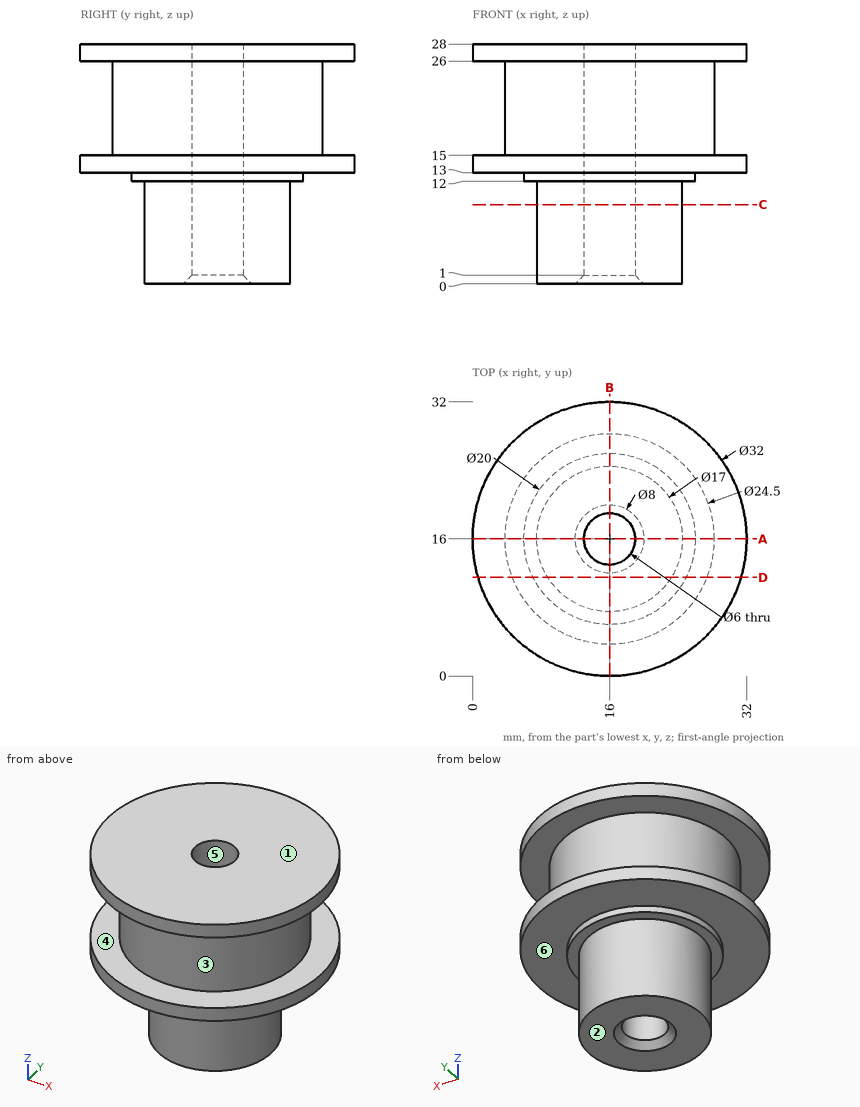
Part print with two shaded views. Sizes in mm from the minimum x, y, z corner. A direction names the side the tool comes from. Give positions to 0.01 mm unless a question says otherwise; leave off trailing zeros. Loops run counter-clockwise (first coordinate to the right, second up) from the corner with the lowest first, then second, coordinate; pieces in that order, holes last. Notation, with made-up numbers: (70, 19) - (78, 19) arc R25 cw to (78, 42) - close; hole circle Ø5 at (52, 23). An arc over 180 degrees is marked (long way). Put each result on its own line as item: value.
Q1. Mould opens along Z. For the marked faces 1, 2 and 3 say: pulls with the +Z half, pulls with the -Z half, needs draft (parallel to the pull), parting line crosses it, or undercut.
Filled in:
face 1: pulls with the +Z half
face 2: pulls with the -Z half
face 3: undercut
Q2. Tool access for the marked faces 4, 5 and 6: list every direction of +Z, -Z, +X, -X, +Y, -Y with a clear straight run to the whole face (end or side of a thin tool).
Filled in:
face 4: none
face 5: +Z, -Z
face 6: -Z
Q3. Probe line 1 along Y through (x, z) = (16, 17.5); line 2 along Z through (x, y) = (27.5, 25); line 3 along X through (y, z) = (17, 2). List the from-to ranges inside material, lowest first.
Filled in:
line 1: y = 3.75 to 13, 19 to 28.25
line 2: z = 13 to 15, 26 to 28
line 3: x = 7.56 to 13.17, 18.83 to 24.44
Q4. Slice it at A-A (y = 16). Give the cut face in (x, z).
Filled in:
outline: (0, 13) - (6, 13) - (6, 12) - (7.5, 12) - (7.5, 0) - (12, 0) - (13, 1) - (13, 28) - (0, 28) - (0, 26) - (3.75, 26) - (3.75, 15) - (0, 15) - close; (19, 1) - (20, 0) - (24.5, 0) - (24.5, 12) - (26, 12) - (26, 13) - (32, 13) - (32, 15) - (28.25, 15) - (28.25, 26) - (32, 26) - (32, 28) - (19, 28) - close
Q5. Flat gauge pins, fed straight in: pin 1 (1.5 mm diameter, centred on x = 16.5, z = 11.5, fed in from -Y); pin 2 (2 mm diameter, centred on y = 19.5, z = 3.5, fed in from +X); pin 3 (4 mm diameter, centred on x = 15, z = 4.5, fed in from +Y); pin 4 (3.5 mm diameter, centred on x = 16, y = 16, fed in from +Z). Where does each tip first touch, or does it go through?
Filled in:
pin 1: stops at y = 6
pin 2: stops at x = 24.12
pin 3: stops at y = 24.5
pin 4: passes through
Q6. Slice it at D-D (y = 11.5). Give the cut face in (x, z).
Filled in:
outline: (0.65, 13) - (7.07, 13) - (7.07, 12) - (8.79, 12) - (8.79, 0) - (23.21, 0) - (23.21, 12) - (24.93, 12) - (24.93, 13) - (31.35, 13) - (31.35, 15) - (27.39, 15) - (27.39, 26) - (31.35, 26) - (31.35, 28) - (0.65, 28) - (0.65, 26) - (4.61, 26) - (4.61, 15) - (0.65, 15) - close
Q7. Slice it at C-C (z = 9.25). Give the cut face in (x, y).
Filled in:
outline: circle Ø17 at (16, 16); hole circle Ø6 at (16, 16)
